Work out the finished part from the listing and answer in its coordinate system (mm). Face numbers are marked on the shaded views. A direction names the side the tool comes from. Give positions to 0.01 mm unless a question says otherwise; leave off trailing zeros. Write each loop counter-clockwise with the first axis right and the second up, starting at its lowest first coordinate (ties: lowest second). Pieces come first, ordered by that corner, then holes. Notation, with made-up numbers: (72, 16) -> (86, 16) arc R13 ccw to (86, 28) -> close; hole circle Ø1 at (35, 87.25). An arc over 180 degrees is marked (long way). Use a Markdown table: item, result. Add a question column.
Q1. For the marked faces 1 and 2, determine the directions among +Z, -Z, +X, -X, +Y, -Y from which every point of the face is accessible in a straight line to the end or side of a thin tool.
Q2. Each of these flat-tipped pins is pushed along its axis until it touches: pin 1 Ø1 at (x, y) = (148.5, 23) entering from -Z; pin 2 Ø14.5 at (y, z) = (31.5, 93.5) entering from -X; pin 3 Ø6 at (x, z) = (67, 45.5) entering from +Y. Where does it stop, or does it pass through?
Q3. Consider line 1 (X direction, y = 29, z = 125.5); line 2 (Y direction, x = 67, z = 93.5); line 3 (Z direction, x = 447.5, y = 44.5). Determine where each line is inside the solid, lowest interval first.
Q4. Section A-A, the plane z = 89 is taken. Give the vertices of the cut face in (x, y) (3 decimals), plus the area to 3 significant figures.
Q5. Section B-B, the plane x = 157 is taken. Give the vertices of the cut face in (y, z) (3 decimals), plus the area to 3 significant figures.
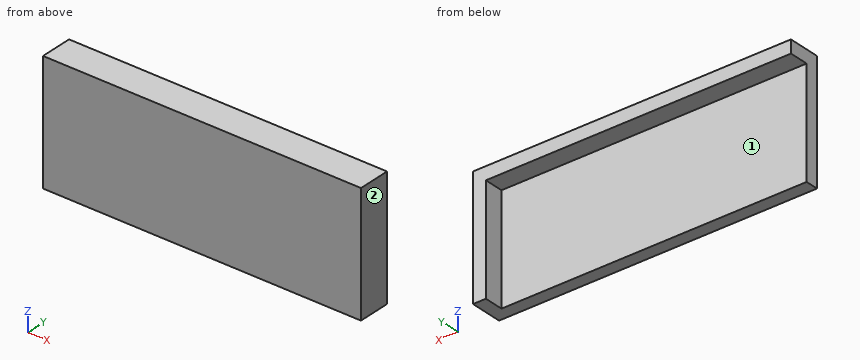
from build123d import *

# Parameters (mm, degrees)
F0_W     = 469.9
F0_H     = 177.8
F1_DEPTH = 19.05
F3_DEPTH = 28.575


with BuildPart() as f1:
    # F0 (on Front) → F1 (new body)
    with BuildSketch(Plane.XZ):
        with Locations((234.95, 88.9)):
            Rectangle(F0_W, F0_H)
    extrude(amount=-F1_DEPTH)

    # F2 (on face) → F3 (join)
    with BuildSketch(Plane(origin=(0, 19.05, 0), x_dir=(-1, 0, 0), z_dir=(0, 1, 0))):
        Polygon((-469.9, 177.8), (-469.9, 0), (-450.85, 0), (-450.85, 158.75), (0, 158.75), (0, 177.8), align=None)
    extrude(amount=F3_DEPTH)


solid = f1.part
Result set:
| question | item | result |
|---|---|---|
| 1 | face 1 | -Z, -X, +Y |
| 1 | face 2 | +Z, -Z, +X, +Y, -Y |
| 2 | pin 1 | stops at z = 158.75 |
| 2 | pin 2 | stops at x = 450.85 |
| 2 | pin 3 | stops at y = 19.05 |
| 3 | line 1 | x = 450.85 to 469.9 |
| 3 | line 2 | y = 0 to 19.05 |
| 3 | line 3 | z = 158.75 to 177.8 |
| 4 | outline | (0, 0) -> (469.9, 0) -> (469.9, 47.625) -> (450.85, 47.625) -> (450.85, 19.05) -> (0, 19.05) -> close |
| 4 | area | 9,500 mm2 |
| 5 | outline | (0, 0) -> (19.05, 0) -> (19.05, 158.75) -> (47.625, 158.75) -> (47.625, 177.8) -> (0, 177.8) -> close |
| 5 | area | 3,930 mm2 |
